The model under review builds one solid part; all positions refer to its coordinate system, in mm. A direction names the side the tool comes from. Give positions to 0.01 mm unless a question says otherwise; leave off trailing zeros. Order: outer loops, then holes, each group sorted by start corner. A loop starts at its lowest first (then second) coordinate and runs counter-clockwise, first axis right, second up. Notation, with made-up numbers: (78, 56) -> (112, 56) arc R14 ccw to (112, 68) -> close; hole circle Ø11 at (-27, 78). An arc over 180 degrees is marked (long way). Use one line per item in the form item = value.
```python
from build123d import *

# Parameters (mm, degrees)
SKETCH1_R           = 17.5
BOSS_EXTRUDE1_DEPTH = 45
SKETCH7_R           = 1.75
BOSS_EXTRUDE2_DEPTH = 5


with BuildPart() as part:
    # Sketch1 → Boss-Extrude1 (new body)
    with BuildSketch(Plane.XY.offset(33.02)):
        Circle(SKETCH1_R)
    extrude(amount=-BOSS_EXTRUDE1_DEPTH)

    # Sketch6 → Revolve5 (revolve)
    with BuildSketch(Plane(origin=(0, 0, 0), x_dir=(1, 0, 0), z_dir=(0, 1, 0))):
        Polygon((5, -33.02), (0, -33.02), (0, -51.02), (2.5, -51.02), (2.5, -37.72), (5, -37.72), align=None)
    revolve(axis=Axis((0, 0, 33.02), (0, 0, 1)))

    # Sketch7 → Boss-Extrude2 (add)
    with BuildSketch(Plane.XY.offset(33.02)):
        with BuildLine():
            Line((17.12018182, 3.626206621), (20.583916427, 3.626206621))
            ThreePointArc((20.583916427, 3.626206621), (23.906641712, 2.207698792), (24.381596036, -1.373793379))
            Line((24.381596036, -1.373793379), (15.366508532, -8.373793379))
            Line((15.366508532, -8.373793379), (17.12018182, 3.626206621))
        make_face()
        with Locations((21, 0)):
            Circle(SKETCH7_R, mode=Mode.SUBTRACT)
        with BuildLine():
            Line((-17.12018182, 3.626206621), (-20.583916427, 3.626206621))
            ThreePointArc((-20.583916427, 3.626206621), (-23.906641712, 2.207698792), (-24.381596036, -1.373793379))
            Line((-24.381596036, -1.373793379), (-15.366508532, -8.373793379))
            Line((-15.366508532, -8.373793379), (-17.12018182, 3.626206621))
        make_face()
        with Locations((-21, 0)):
            Circle(SKETCH7_R, mode=Mode.SUBTRACT)
    extrude(amount=-BOSS_EXTRUDE2_DEPTH)


solid = part.part
```
1. For pin 1 Ø3 at (x, y) = (-21.5, -4.5) entering from -Z; pin 2 Ø6 at (x, z) = (15.5, 23.5) entering from -Y; pin 3 Ø10 at (y, z) = (2, 19.5) entering from -X, all flat-tipped, find the tip position at first contact; note any pin that passes through.
Values:
pin_1 = 28.02
pin_2 = -12.25
pin_3 = -17.5
2. The part is to be moulded in two halves that separate along Y. For faces 1 (the face through (23.874, 2.25, 30.555)), 2 (the face through (19, -1, 28.02)), 3 (the face through (19.25, 0.08, 30.56)), say which applies: +Y half, -Y half, draft (parallel to the pull), parting line (faces both ways), or undercut.
Values:
face_1 = parting line
face_2 = draft
face_3 = undercut
3. Add section B-B on x = 0. Give the boundary of the cut face in (y, z), then the cut area to 3 significant figures.
Values:
outline = (-17.5, -11.98) -> (17.5, -11.98) -> (17.5, 33.02) -> (5, 33.02) -> (5, 37.72) -> (2.5, 37.72) -> (2.5, 51.02) -> (-2.5, 51.02) -> (-2.5, 37.72) -> (-5, 37.72) -> (-5, 33.02) -> (-17.5, 33.02) -> close
area = 1,690 mm^2
4. Add section A-A on y = 0. Give the boundary of the cut face in (x, z).
Values:
outline = (-24.65, 28.02) -> (-22.75, 28.02) -> (-22.75, 33.02) -> (-24.65, 33.02) -> close; (-19.25, 28.02) -> (-17.5, 28.02) -> (-17.5, -11.98) -> (17.5, -11.98) -> (17.5, 28.02) -> (19.25, 28.02) -> (19.25, 33.02) -> (5, 33.02) -> (5, 37.72) -> (2.5, 37.72) -> (2.5, 51.02) -> (-2.5, 51.02) -> (-2.5, 37.72) -> (-5, 37.72) -> (-5, 33.02) -> (-19.25, 33.02) -> close; (22.75, 28.02) -> (24.65, 28.02) -> (24.65, 33.02) -> (22.75, 33.02) -> close
5. For L1, parallel to Z at x = 7.5, y = 11; L2, parallel to Y at x = 21, z = 29.25; L3, parallel to Y at x = 20, z = 31.5, list the stretches that pass through material, from the lowest coordinate up.
Values:
L1 = -11.98 to 33.02
L2 = -4 to -1.75, 1.75 to 3.65
L3 = -4.78 to -1.44, 1.44 to 3.63
6. Add section C-C on z = 39.5. Give the boundary of the cut face in (x, y), then the cut area to 3 significant figures.
Values:
outline = circle Ø5 at (0, 0)
area = 19.6 mm^2
7. Add section D-D on y = -15. Give the boundary of the cut face in (x, z), then the cut area to 3 significant figures.
Values:
outline = (-9.01, -11.98) -> (9.01, -11.98) -> (9.01, 33.02) -> (-9.01, 33.02) -> close
area = 811 mm^2
8. Tool access review of faces 4 (the face through (-1.08, -4.88, 35.34)), 5 (the face through (9.408, 14.756, 10.835)): name each direction out of +Z, -Z, +X, -X, +Y, -Y from which nothing blocks a thin tool from reaching the whole face with its end or side.
Values:
face_4 = +Z
face_5 = -Z
